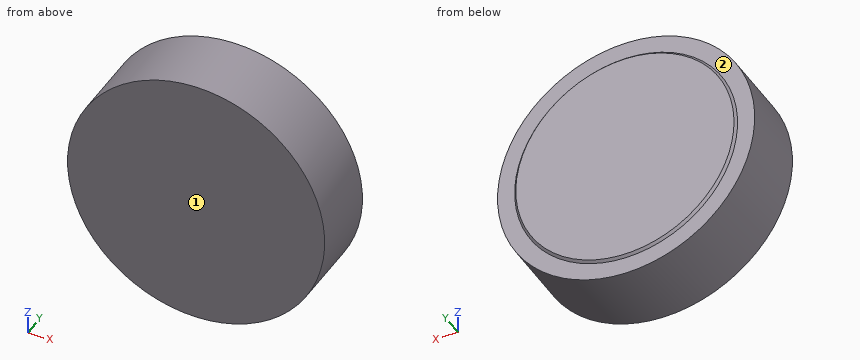
from build123d import *

# Parameters (mm, degrees)
SKETCH1_R           = 5.5
BOSS_EXTRUDE1_DEPTH = 3.1
SKETCH2_R           = 5.167835257
BOSS_EXTRUDE2_DEPTH = 0.1
CHAMFER1_SIZE       = 0.5


with BuildPart() as part:
    # Sketch1 → Boss-Extrude1 (new body)
    with BuildSketch(Plane(origin=(0, 0, 0), x_dir=(1, 0, 0), z_dir=(0, 1, 0))):
        with Locations(Location((0, 0, 0), (0, 0, 90))):
            Circle(SKETCH1_R)
    extrude(amount=BOSS_EXTRUDE1_DEPTH)

    # Sketch2 → Boss-Extrude2 (add)
    with BuildSketch(Plane(origin=(0, 3.1, 0), x_dir=(1, 0, 0), z_dir=(0, 1, 0))):
        with Locations(Location((0, 0, 0), (0, 0, 270))):
            Circle(SKETCH2_R)
    extrude(amount=BOSS_EXTRUDE2_DEPTH)

    # Chamfer1
    # the kernel refuses this chamfer: 0.5 mm, written as the material it takes off along each edge
    with BuildSketch(Plane(origin=(0, 3.2, 0), x_dir=(0, 0, 1), z_dir=(-1, 0, 0))) as chamfer1_piece_1_section:
        Polygon((5.167835257, -CHAMFER1_SIZE), (5.167835257 - CHAMFER1_SIZE, 0), (5.167835257, 0), align=None)
    chamfer1_piece_1 = revolve(axis=Axis((0, 3.2, 0), (0, 1, 0)), mode=Mode.PRIVATE)
    chamfer1_piece_1 = split(chamfer1_piece_1, bisect_by=Plane(origin=(0, 3.1, -4.719067591), z_dir=(0, 1, 0)), keep=Keep.TOP, mode=Mode.PRIVATE)
    add(chamfer1_piece_1, mode=Mode.SUBTRACT)


solid = part.part
For this review, take the finished solid that the model builds, in its own axes (mm). Face numbers are marked on the shaded views. A direction names the side the tool comes from. Round coordinates to 2 decimals unless told otherwise and drop trailing zeros. Write each loop counter-clockwise with the first axis right and the second up, starting at its lowest first coordinate (ties: lowest second). Pieces come first, ordered by that corner, then holes. Notation, with made-up numbers: (-6.5, -36) - (47.5, -36) arc R24 cw to (47.5, 1) - close; hole circle Ø2 at (-24, 86.25). An arc over 180 degrees is marked (long way). Write item = value, one per line. Start each with the question number.
1. Consider section A-A on y = 1.75. State the section outline as (x, z) points.
2. For the marked faces 1 and 2, list the 3-axis set-ups (+Z, -Z, +X, -X, +Y, -Y) from which the entire face can be reached by the end or side of a thin tool; tool diameter is ignored.
3. Wall thickness on L1, parallel to Y at x = -3, z = -4.5; L2, parallel to X at y = 2.55, z = 1.5; L3, parallel to Z at x = 2, y = 3.05: over which ranges is each line inside the solid? List them lowest first.
Evaluation:
q1.outline = circle Ø11 at (0, 0)
q2.face_1 = +Z, -Z, +X, -X, -Y
q2.face_2 = +Y
q3.L1 = 0 to 3.1
q3.L2 = -5.29 to 5.29
q3.L3 = -5.12 to 5.12
